Autodesk Inventor part; units mm, degrees
ref_plane "YZ Plane" through (0, 0, 0) normal (1, 0, 0) x (0, 1, 0)
ref_plane "XZ Plane" through (0, 0, 0) normal (0, 1, 0) x (-1, 0, 0)
ref_plane "XY Plane" through (0, 0, 0) normal (0, 0, 1) x (1, 0, 0)
sketch "Sketch1" plane through (0, 0, 0) normal (0, 0, 1) x (1, 0, 0)
  arc A0 (-2.2, 21.8897) -> (-21.8897, 2.2) centre (0, 0) ccw
  line L0 (-11.05, 0) -> (-19.8997, 0)
  line L1 (0, 11.05) -> (0, 19.8997)
  line L2 (0, 0) -> (22, 0) construction
  circle A1 centre (-12.1976, 12.1976) radius 2.8
  line L3 (0.5858, 7.4045) -> (6.9261, 1.0642)
  arc A2 (-21.8897, 2.2) -> (-19.8997, 0) centre (-19.8997, 2) ccw
  arc A3 (0, 19.8997) -> (-2.2, 21.8897) centre (-2, 19.8997) ccw
  line L4 (-8.5302, 2.5198) -> (-9.2373, 3.2269)
  line L5 (-3.2269, 9.2373) -> (-2.5198, 8.5302)
  line L6 (-0.1156, -5.8948) -> (-8.5302, 2.5198)
  line L7 (-2.5198, 8.5302) -> (5.8948, 0.1156)
  line L8 (-11.05, 0) -> (-8.8187, 0)
  line L9 (-7.4045, -0.5858) -> (-1.0642, -6.9261)
  line L10 (0, 11.05) -> (0, 8.8187)
  arc A4 (-7.4045, -0.5858) -> (-8.8187, 0) centre (-8.8187, -2) ccw
  arc A5 (0, 8.8187) -> (0.5858, 7.4045) centre (2, 8.8187) ccw
  arc A6 (0, 11.05) -> (-1.5191, 10.9451) centre (0, 0) ccw
  line L11 (5.8948, 0.1156) -> (7.309, -1.2986)
  line L12 (-0.1156, -5.8948) -> (1.2986, -7.309)
  line L13 (-0.1156, -5.8948) -> (1.8844, -5.8948) construction
  line L14 (1.2986, -7.309) -> (7.309, -1.2986)
  line L15 (-9.2373, 3.2269) -> (-3.2269, 9.2373)
  line L16 (-1.0642, -6.9261) -> (-0.1156, -7.8747)
  line L17 (2.7128, -7.8747) -> (7.8747, -2.7128)
  line L18 (7.8747, 0.1156) -> (6.9261, 1.0642)
  arc A7 (-10.2177, 4.2073) -> (-10.7101, 2.7198) centre (0, 0) ccw
  arc A8 (-10.9451, 1.5191) -> (-11.05, 0) centre (0, 0) ccw
  arc A9 (7.8747, -2.7128) -> (7.8747, 0.1156) centre (6.4605, -1.2986) ccw
  arc A10 (-0.1156, -7.8747) -> (2.7128, -7.8747) centre (1.2986, -6.4605) ccw
  point P0 (-22, 0)
  point P1 (0, 22)
  point P2 (0, 7.9903)
  point P3 (-4.2073, 10.2177)
  dimension "d1" = 44
  dimension "d3" = 5.6
  dimension "d4" = 17.25
  dimension "d6" = 15.6271
  dimension "d16" = 1
  dimension "d18" = 2
  dimension "d19" = 1
  dimension "d20" = 2
  dimension "d21" = 2
  dimension "d22" = 45
  dimension "d23" = 14.9
  dimension "d24" = 2
extrude "Extrusion1" add sketch "Sketch1" along normal blind 2.4
properties part number "ir-holder"
Can you work these out from the model? Positions are in its coordinate system, mm. A direction names the side the tool comes from. Give positions to 0.01 mm unless a question says otherwise; leave off trailing zeros. Write each loop counter-clockwise with the first axis right and the second up, starting at its lowest first coordinate (ties: lowest second). Pieces come first, ordered by that corner, then holes. Notation, with made-up numbers: (27.5, -10) -> (42.5, -10) arc R24 ccw to (42.5, 14) -> close; hole circle Ø8 at (-32.5, 8.25). An arc over 180 degrees is marked (long way). One line per item, written item: value.
Q1. Which directions (+Z, -Z, +X, -X, +Y, -Y) give clear straight access to the entire face, cutting with the end or side of a thin tool? Please do faces 5 (the face through (-14, 0, 1)), 6 (the face through (0, 14, 1)), 7 (the face through (1.97, 4.04, 1.18)).
Results found:
face 5: +Z, -Z, -X, -Y
face 6: +Z, -Z, +X, +Y
face 7: +Z, -Z
Q2. Imagine slicing it at B-B on y = 13.5. Please give me the cut outline in (x, z).
Results found:
outline: (-17.37, 0) -> (-14.68, 0) -> (-14.68, 2.4) -> (-17.37, 2.4) -> close; (-9.72, 0) -> (0, 0) -> (0, 2.4) -> (-9.72, 2.4) -> close
Q3. Please list where these lines run through material, in increasing order: line 1 (X direction, y = -7, z = 1.1); line 2 (Y direction, x = -10.5, z = 1.3); line 3 (Y direction, x = -0.5, z = 0.9). Write a range as [from, to].
Results found:
line 1: x = [-0.99, 0.99], [1.61, 3.59]
line 2: y = [0, 9.97], [14.42, 19.33]
line 3: y = [-7.49, -5.51], [6.51, 21.22]
Q4. We'd pull the mould along Y, two halves only. Please class faces 1 (the face through (4.26, -4.35, 1.18)), 2 (the face through (-7, 7, 0)), 3 (the face through (-6.274, 6.19, 1.183)), 4 (the face through (4.28, 3.71, 1.18)): +Y half, -Y half, draft (parallel to the pull), parting line (faces both ways), or undercut.
Results found:
face 1: undercut
face 2: draft
face 3: undercut
face 4: +Y half
Q5. Imagine slicing it at C-C on z = 0.45. Please give me the cut outline in (x, y).
Results found:
outline: (-21.89, 2.2) arc R2 ccw to (-19.9, 0) -> (-8.82, 0) arc R2 cw to (-7.4, -0.59) -> (-0.12, -7.87) arc R2 ccw to (2.71, -7.87) -> (7.87, -2.71) arc R2 ccw to (7.87, 0.12) -> (0.59, 7.4) arc R2 cw to (0, 8.82) -> (0, 19.9) arc R2 ccw to (-2.2, 21.89) arc R22 ccw to start; hole circle Ø5.6 at (-12.2, 12.2); hole (-9.24, 3.23) -> (1.3, -7.31) -> (7.31, -1.3) -> (-3.23, 9.24) -> close
Q6. For P1, Ø0.7, axis at y = 17, z = 1, coming from the +X side; P2, Ø1, axis at y = 4.5, z = 1.5, coming from the +X side, each with a flat end and sliding along its axis, tell me the tip position at first contact or that it passes through.
Results found:
P1: stops at x = 0
P2: stops at x = 3.99
Q7. Imagine slicing it at A-A on x = -0.5. Please give me the cut outline in (y, z).
Results found:
outline: (-7.49, 0) -> (-5.51, 0) -> (-5.51, 2.4) -> (-7.49, 2.4) -> close; (6.51, 0) -> (21.22, 0) -> (21.22, 2.4) -> (6.51, 2.4) -> close
